```python
from build123d import *

# Parameters (mm, degrees)
SKETCH_1_W          = 154
SKETCH_1_H          = 50
EXTRUDE_1_DEPTH     = 2
SKETCH_2_R          = 1
CUT_EXTRUDE_1_DEPTH = 10
CUT_EXTRUDE_2_DEPTH = 10
SKETCH_4_R          = 1.5
CUT_EXTRUDE_3_DEPTH = 10
FILLET_1_R          = 3
CUT_EXTRUDE_4_DEPTH = 5
SKETCH_6_R          = 3
SKETCH_6_R_2        = 1
EXTRUDE_2_DEPTH     = 2
FILLET_2_R          = 2
CUT_EXTRUDE_5_DEPTH = 5
FILLET_3_R          = 4
FILLET_4_R          = 2
SKETCH_19_R         = 1.5
CUT_EXTRUDE_6_DEPTH = 10
SKETCH_20_R         = 1.5
CUT_EXTRUDE_7_DEPTH = 81.981479493
SKETCH_22_R         = 1.2
CUT_EXTRUDE_9_DEPTH = 10


with BuildPart() as part:
    # 草图1 → 凸台-拉伸1 (new body)
    with BuildSketch(Plane.XY):
        Rectangle(SKETCH_1_W, SKETCH_1_H)
    extrude(amount=EXTRUDE_1_DEPTH)

    # 草图2 → 切除-拉伸1 (cut)
    with BuildSketch(Plane(origin=(0, 0, 0), x_dir=(-1, 0, 0), z_dir=(0, 0, -1))):
        with Locations((22.6, 9)):
            Circle(SKETCH_2_R)
        with Locations(Location((-22.6, 9, 0), (0, 0, 180))):
            Circle(SKETCH_2_R)
        with Locations(Location((22.6, -9, 0), (0, 0, 180))):
            Circle(SKETCH_2_R)
        with Locations((-22.6, -9)):
            Circle(SKETCH_2_R)
    extrude(amount=-CUT_EXTRUDE_1_DEPTH, mode=Mode.SUBTRACT)

    # 草图3 → 切除-拉伸2 (cut)
    with BuildSketch(Plane.XY.offset(2)):
        Polygon((-77, -25), (-48, 25), (-77, 25), align=None)
    extrude(amount=-CUT_EXTRUDE_2_DEPTH, mode=Mode.SUBTRACT)

    # 草图4 → 切除-拉伸3 (cut)
    with BuildSketch(Plane(origin=(0, 0, 0), x_dir=(-1, 0, 0), z_dir=(0, 0, -1))):
        with Locations((-42, -22)):
            Circle(SKETCH_4_R)
        with Locations((-17, -22)):
            Circle(SKETCH_4_R)
        with Locations((8, -22)):
            Circle(SKETCH_4_R)
        with Locations((33, -22)):
            Circle(SKETCH_4_R)
        with Locations((58, -22)):
            Circle(SKETCH_4_R)
    extrude(amount=-CUT_EXTRUDE_3_DEPTH, mode=Mode.SUBTRACT)

    # 圆角1
    fillet_1_edges = [part.edges().sort_by_distance(p)[0] for p in [
        (-48, 25, 1),
        (77, 25, 1),
        (77, -25, 1),
        (-77, -25, 1),
    ]]
    fillet(fillet_1_edges, radius=FILLET_1_R)

    # 草图5 → 切除-拉伸4 (cut)
    with BuildSketch(Plane(origin=(0, 0, 0), x_dir=(-1, 0, 0), z_dir=(0, 0, -1))):
        with BuildLine():
            Line((4.06564659, -14.982340198), (-10.985896104, 10.96859548))
            ThreePointArc((-10.985896104, 10.96859548), (-9.532643706, 16.435592596), (-4.06564659, 14.982340198))
            Line((-4.06564659, 14.982340198), (10.985896104, -10.96859548))
            ThreePointArc((10.985896104, -10.96859548), (9.532643706, -16.435592596), (4.06564659, -14.982340198))
        make_face()
        with BuildLine():
            Line((20.06564659, -14.982340198), (5.014103896, 10.96859548))
            ThreePointArc((5.014103896, 10.96859548), (6.467356294, 16.435592596), (11.93435341, 14.982340198))
            Line((11.93435341, 14.982340198), (26.985896104, -10.96859548))
            ThreePointArc((26.985896104, -10.96859548), (25.532643706, -16.435592596), (20.06564659, -14.982340198))
        make_face()
        with BuildLine():
            Line((36.06564659, -14.982340198), (21.014103896, 10.96859548))
            ThreePointArc((21.014103896, 10.96859548), (22.467356294, 16.435592596), (27.93435341, 14.982340198))
            Line((27.93435341, 14.982340198), (42.985896104, -10.96859548))
            ThreePointArc((42.985896104, -10.96859548), (41.532643706, -16.435592596), (36.06564659, -14.982340198))
        make_face()
        with BuildLine():
            Line((52.06564659, -14.982340198), (37.014103896, 10.96859548))
            ThreePointArc((37.014103896, 10.96859548), (38.467356294, 16.435592596), (43.93435341, 14.982340198))
            Line((43.93435341, 14.982340198), (58.985896104, -10.96859548))
            ThreePointArc((58.985896104, -10.96859548), (57.532643706, -16.435592596), (52.06564659, -14.982340198))
        make_face()
        with BuildLine():
            Line((-11.93435341, -14.982340198), (-26.985896104, 10.96859548))
            ThreePointArc((-26.985896104, 10.96859548), (-25.532643706, 16.435592596), (-20.06564659, 14.982340198))
            Line((-20.06564659, 14.982340198), (-5.014103896, -10.96859548))
            ThreePointArc((-5.014103896, -10.96859548), (-6.467356294, -16.435592596), (-11.93435341, -14.982340198))
        make_face()
        with BuildLine():
            Line((-27.93435341, -14.982340198), (-42.985896104, 10.96859548))
            ThreePointArc((-42.985896104, 10.96859548), (-41.532643706, 16.435592596), (-36.06564659, 14.982340198))
            Line((-36.06564659, 14.982340198), (-21.014103896, -10.96859548))
            ThreePointArc((-21.014103896, -10.96859548), (-22.467356294, -16.435592596), (-27.93435341, -14.982340198))
        make_face()
        with BuildLine():
            Line((-43.93435341, -14.982340198), (-58.985896104, 10.96859548))
            ThreePointArc((-58.985896104, 10.96859548), (-57.532643706, 16.435592596), (-52.06564659, 14.982340198))
            Line((-52.06564659, 14.982340198), (-37.014103896, -10.96859548))
            ThreePointArc((-37.014103896, -10.96859548), (-38.467356294, -16.435592596), (-43.93435341, -14.982340198))
        make_face()
    extrude(amount=-CUT_EXTRUDE_4_DEPTH, mode=Mode.SUBTRACT)

    # 草图6 → 凸台-拉伸2 (add)
    # profile 1 of 4: a face of its own
    with BuildSketch(Plane(origin=(0, 0, 0), x_dir=(-1, 0, 0), z_dir=(0, 0, -1))):
        with Locations((22.6, 9)):
            Circle(SKETCH_6_R)
        with Locations((22.6, 9)):
            Circle(SKETCH_6_R_2, mode=Mode.SUBTRACT)
    # profile 2 of 4: a face of its own
    with BuildSketch(Plane(origin=(0, 0, 0), x_dir=(-1, 0, 0), z_dir=(0, 0, -1))):
        with Locations((22.6, -9)):
            Circle(SKETCH_6_R)
        with Locations((22.6, -9)):
            Circle(SKETCH_6_R_2, mode=Mode.SUBTRACT)
    # profile 3 of 4: a face of its own
    with BuildSketch(Plane(origin=(0, 0, 0), x_dir=(-1, 0, 0), z_dir=(0, 0, -1))):
        with Locations((-22.6, -9)):
            Circle(SKETCH_6_R)
        with Locations((-22.6, -9)):
            Circle(SKETCH_6_R_2, mode=Mode.SUBTRACT)
    # profile 4 of 4: a face of its own
    with BuildSketch(Plane(origin=(0, 0, 0), x_dir=(-1, 0, 0), z_dir=(0, 0, -1))):
        with Locations((-22.6, 9)):
            Circle(SKETCH_6_R)
        with Locations(Location((-22.6, 9, 0), (0, 0, 180))):
            Circle(SKETCH_6_R_2, mode=Mode.SUBTRACT)
    extrude(amount=-EXTRUDE_2_DEPTH)

    # 圆角2
    fillet_2_edges = [part.edges().sort_by_distance(p)[0] for p in [
        (-20.798153142, 11.398613745, 1),
        (-23.760443426, 6.233527326, 1),
        (-24.495365876, -6.674577845, 1),
        (-25.559633713, -8.509522393, 1),
        (20.798153142, -11.398613745, 1),
        (23.760443426, -6.233527326, 1),
        (24.495365876, 6.674577845, 1),
        (25.559633713, 8.509522393, 1),
    ]]
    fillet(fillet_2_edges, radius=FILLET_2_R)

    # 草图7 → 切除-拉伸5 (cut)
    with BuildSketch(Plane(origin=(0, 0, 0), x_dir=(-1, 0, 0), z_dir=(0, 0, -1))):
        Polygon((-68.8095376, 11.960699007), (-52.026560829, -16.975467839), (-68.8095376, -16.975467839), align=None)
    extrude(amount=-CUT_EXTRUDE_5_DEPTH, mode=Mode.SUBTRACT)

    # 圆角3
    fillet_3_edges = [part.edges().sort_by_distance(p)[0] for p in [
        (52.026560829, -16.975467839, 1),
        (68.8095376, -16.975467839, 1),
    ]]
    fillet(fillet_3_edges, radius=FILLET_3_R)

    # 圆角4
    fillet_4_edges = [part.edges().sort_by_distance(p)[0] for p in [
        (68.8095376, 11.960699007, 1),
    ]]
    fillet(fillet_4_edges, radius=FILLET_4_R)

    # 草图19 → 切除-拉伸6 (cut)
    with BuildSketch(Plane(origin=(0, 0, 0), x_dir=(-1, 0, 0), z_dir=(0, 0, -1))):
        with Locations((-74, -13)):
            Circle(SKETCH_19_R)
        with Locations((-74, 7)):
            Circle(SKETCH_19_R)
    extrude(amount=-CUT_EXTRUDE_6_DEPTH, mode=Mode.SUBTRACT)

    # 草图20 → 切除-拉伸7 (cut, through all)
    with BuildSketch(Plane(origin=(0, 0, 0), x_dir=(-1, 0, 0), z_dir=(0, 0, -1))):
        with Locations((64.219334799, -8.943823867)):
            Circle(SKETCH_20_R)
        with Locations((54.184973003, 8.356799919)):
            Circle(SKETCH_20_R)
    extrude(amount=-CUT_EXTRUDE_7_DEPTH, mode=Mode.SUBTRACT)

    # 草图22 → 切除-拉伸9 (cut)
    with BuildSketch(Plane(origin=(0, 0, 0), x_dir=(-1, 0, 0), z_dir=(0, 0, -1))):
        with Locations((-41.62550176, 22)):
            Circle(SKETCH_22_R)
        with Locations((-61.62550176, 22)):
            Circle(SKETCH_22_R)
    extrude(amount=-CUT_EXTRUDE_9_DEPTH, mode=Mode.SUBTRACT)


solid = part.part
```
Work out the finished part from the listing and answer in its coordinate system (mm). Give positions to 0.01 mm unless a question says otherwise; leave off trailing zeros. Order: outer loops, then holes, each group sorted by start corner. A loop starts at its lowest first (then second) coordinate and runs counter-clockwise, first axis right, second up.
1. Section A-A, the plane x = 17 is taken. Determine the outline of the cut face in (y, z), and give its area (3 significant figures).
Result sheet:
outline: (-25, 0) - (-23.5, 0) - (-23.5, 2) - (-25, 2) - close; (-20.5, 0) - (-6.25, 0) - (-6.25, 2) - (-20.5, 2) - close; (9.7, 0) - (25, 0) - (25, 2) - (9.7, 2) - close
area: 62.1 mm2
2. Each of these flat-tipped pins is pushed along its axis until it touches: P1, Ø2.5, axis at x = 22.6, y = 9, coming from the +Z side; P2, Ø1, axis at y = -3, z = 0.5, coming from the -X side. Where does it stop, or does it pass through?
Result sheet:
P1: stops at z = 2
P2: stops at x = -64.53
3. Straight lines are drawn through the part: L1, parallel to Y at x = -37, z = 1.9; L2, parallel to Y at x = -54, z = 0.4; L3, parallel to Y at x = -8, z = 1.4. For each, find the intervals that lie inside material, in ascending order.
Result sheet:
L1: y = -25 to -16.08, -0.65 to 10.99, 14.96 to 25
L2: y = -25 to -16.67, -2.37 to 6.87, 9.85 to 14.66
L3: y = -25 to -23.5, -20.5 to -16.95, -5.82 to 5.82, 16.95 to 25
4. Section B-B, the plane y = 2 is taken. Give the number of separate pieces and of enclosed holes in the cut face, and give its area (3 significant figures).
Result sheet:
separate pieces: 9
enclosed holes: 0
area: 136 mm2
